from build123d import *

# Parameters (mm, degrees)
F0_W          = 20
F0_H          = 15
F1_DEPTH      = 80
F3_DEPTH      = 25
F3_DEPTH_BACK = 5
F4_W          = 12.7
F4_H          = 10
F5_DEPTH      = 8.382
F6_R          = 5
F7_DEPTH      = 25.4


with BuildPart() as f1:
    # F0 (on Right) → F1 (new body)
    with BuildSketch(Plane.YZ):
        with Locations((-33.5142107308, -19.1700014472)):
            Rectangle(F0_W, F0_H)
    extrude(amount=F1_DEPTH)

    # F2 (on face) → F3 (join, two sides)
    with BuildSketch(Plane.XZ.offset(43.5142107308)) as f3_sk:
        Polygon((20, -26.6700014472), (40, -26.6700014472), (40, 8.3299985528), align=None)
        Polygon((40, 8.3299985528), (40, -26.6700014472), (60, -26.6700014472), align=None)
    extrude(amount=-F3_DEPTH)
    extrude(f3_sk.sketch, amount=F3_DEPTH_BACK)

    # F4 (on Top) → F5 (cut)
    with BuildSketch(Plane.XY):
        with Locations((40, -33.5142107308)):
            Rectangle(F4_W, F4_H)
    extrude(amount=F5_DEPTH, mode=Mode.SUBTRACT)

    # F6 (on face) → F7 (cut)
    with BuildSketch(Plane.XY.offset(-11.6700014472)):
        with Locations((10, -33.5142107308)):
            Circle(F6_R)
        with Locations((70, -33.5142107308)):
            Circle(F6_R)
    extrude(amount=-F7_DEPTH, mode=Mode.SUBTRACT)


solid = f1.part
Design review of the part built by this model. Coordinates are the model's own, in mm. A direction names the side the tool comes from. Coordinates: 2 decimals unless noted, no trailing zeros. Write each loop counter-clockwise with the first axis right and the second up, starting at its lowest first coordinate (ties: lowest second). Pieces come first, ordered by that corner, then holes. Notation, with made-up numbers: (82, 34.5) - (139, 34.5) arc R24 cw to (139, 48.5) - close; hole circle Ø11 at (56, 28). An arc over 180 degrees is marked (long way). One line per item, written item: value.
1) Add section C-C (z = 5.5). State the section outline as (x, y) points.
Answer sheet:
outline: (38.38, -48.51) - (41.62, -48.51) - (41.62, -38.51) - (38.38, -38.51) - close; (38.38, -28.51) - (41.62, -28.51) - (41.62, -18.51) - (38.38, -18.51) - close
2) Add section B-B (y = -37.75). State the section outline as (x, z) points, plus the area to 3 significant figures.
Answer sheet:
outline: (0, -26.67) - (7.34, -26.67) - (7.34, -11.67) - (0, -11.67) - close; (12.66, -26.67) - (67.34, -26.67) - (67.34, -11.67) - (51.43, -11.67) - (44.76, 0) - (35.24, 0) - (28.57, -11.67) - (12.66, -11.67) - close; (72.66, -26.67) - (80, -26.67) - (80, -11.67) - (72.66, -11.67) - close
area: 1,230 mm2
3) Insertion check: pin 1 (4.5 mm diameter, centred on x = 18.5, z = -18.5, fed in from -Y); pin 2 (11.5 mm diameter, centred on x = 70, y = -33.51, fed in from +Z); pin 3 (4.5 mm diameter, centred on x = 73, z = -22.5, fed in from +Y); pin 4 (5 mm diameter, centred on x = 9, z = -8, fed in from -Y). Each pin has a flat end and moves straight along its axis. Give the tip position at first contact, or say it passes through.
Answer sheet:
pin 1: stops at y = -43.51
pin 2: stops at z = -11.67
pin 3: stops at y = -23.51
pin 4: passes through
4) To check wall thickness, follow probe 1 along Y at (x, z) = (70, -18); probe 2 along Z at (x, y) = (70.5, -41.5); probe 3 along Y at (x, z) = (12, -21). State the ranges of each line that lie inside material, in increasing order.
Answer sheet:
probe 1: y = -43.51 to -38.51, -28.51 to -23.51
probe 2: z = -26.67 to -11.67
probe 3: y = -43.51 to -38.1, -28.93 to -23.51
5) For faces 1 (the face through (62, -34, -11.67)), 2 (the face through (69, -23.514, -19)), 3 (the face through (17, -34, -11.67)), 4 (the face through (40, -38.514, 3)), 5 (the face through (11, -43.514, -19)), list the 3-axis set-ups (+Z, -Z, +X, -X, +Y, -Y) from which the entire face can be reached by the end or side of a thin tool; tool diameter is ignored.
Answer sheet:
face 1: +Z, +X, +Y, -Y
face 2: +Z, +X, +Y
face 3: +Z, -X, +Y, -Y
face 4: +Z, +X, -X
face 5: +Z, -X, -Y
6) Mouldability with a two-part tool opening along Y and no side actions: class faces 6 (the face through (69, -43.514, -19)), 7 (the face through (40, -18.514, -13)), 8 (the face through (74.77, -32.01, -19.07)) as +Y half, -Y half, draft (parallel to the pull), parting line (faces both ways), or undercut.
Answer sheet:
face 6: -Y half
face 7: +Y half
face 8: undercut
7) Add section A-A (x = 10). State the section outline as (y, z) points.
Answer sheet:
outline: (-43.51, -26.67) - (-38.51, -26.67) - (-38.51, -11.67) - (-43.51, -11.67) - close; (-28.51, -26.67) - (-23.51, -26.67) - (-23.51, -11.67) - (-28.51, -11.67) - close
8) Add section D-D (z = -15). State the section outline as (x, y) points, plus the area to 3 significant figures.
Answer sheet:
outline: (0, -43.51) - (26.67, -43.51) - (26.67, -48.51) - (53.33, -48.51) - (53.33, -43.51) - (80, -43.51) - (80, -23.51) - (53.33, -23.51) - (53.33, -18.51) - (26.67, -18.51) - (26.67, -23.51) - (0, -23.51) - close; hole circle Ø10 at (10, -33.51); hole circle Ø10 at (70, -33.51)
area: 1,710 mm2
